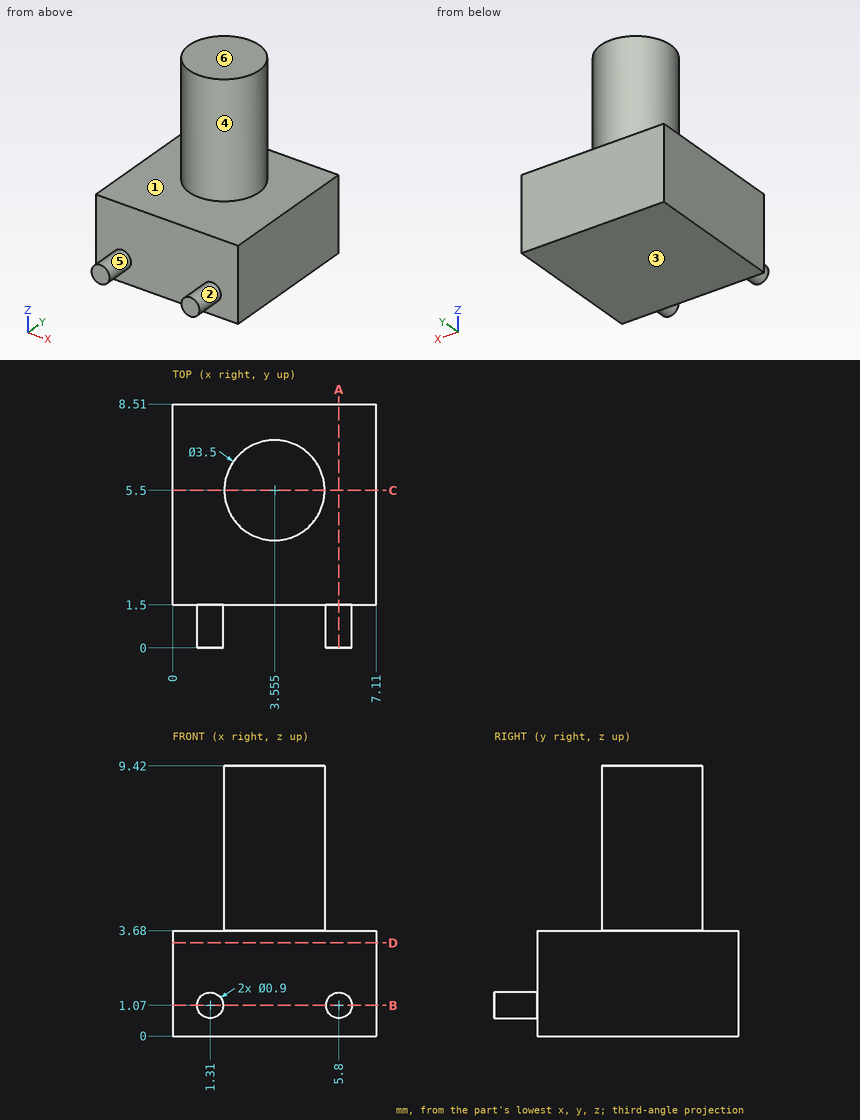
The figure shows three views and two pictorial views of one solid part (mm, origin at its lowest corner). Answer the questions. A direction names the side the tool comes from. Round coordinates to 2 decimals unless told otherwise and drop trailing zeros. Write each loop counter-clockwise with the first axis right and the second up, starting at its lowest first coordinate (ties: lowest second). Pieces come first, ordered by that corner, then holes. Notation, with made-up numbers: M 85.5,45.25 L 120.5,45.25 A16 ccw 120.5,76.25 Z; hole C 59.5,-7 d2. An arc over 180 degrees is marked long. Write each question's results on one line, items separated by ' | '. Start each with the question number.
(1) The part is cut by section A-A, the plane x = 5.8. Write down the section's boundary in (y, z), and give its area (3 significant figures).
(2) The part is cut by section C-C, the plane y = 5.5. Write down the section's boundary in (x, z) (3 decimals).
(3) The part is cut by section B-B, the plane z = 1.07. Write down the section's boundary in (x, y).
(4) The part is cut by section D-D, the plane z = 3.25. Write down the section's boundary in (x, y).
(5) For the marked faces 1, 2 and 3, determine the directions among +Z, -Z, +X, -X, +Y, -Y from which every point of the face is accessible in a straight line to the end or side of a thin tool.
(6) Determine the mould class of the marked faces 4, 5 and 6 for opening direction X: +X half, -X half, draft (parallel to the pull), parting line (faces both ways), or undercut.
(7) Find the intervals of material crossed by line 1 (Z direction, x = 6.75, y = 2); line 2 (X direction, y = 5.5, z = 6.5) (3 decimals); line 3 (Y direction, x = 2.5, z = 6.75), in increasing order.
(8) Each of these flat-tipped pins is pushed along its axis until it touches: P1, Ø2, axis at x = 5.5, y = 3.5, coming from the +Z side; P2, Ø5, axis at y = 5, z = 7, coming from the +X side (3 decimals); P3, Ø3, axis at y = 2.5, z = 7, coming from the -X side. Where does it stop, or does it pass through?
Worked answers:
1) outline: M 0,0.62 L 1.5,0.62 L 1.5,0 L 8.51,0 L 8.51,3.68 L 1.5,3.68 L 1.5,1.52 L 0,1.52 Z | area: 27.1 mm²
2) outline: M 0,0 L 7.11,0 L 7.11,3.68 L 5.305,3.68 L 5.305,9.42 L 1.805,9.42 L 1.805,3.68 L 0,3.68 Z
3) outline: M 0,1.5 L 0.86,1.5 L 0.86,0 L 1.76,0 L 1.76,1.5 L 5.35,1.5 L 5.35,0 L 6.25,0 L 6.25,1.5 L 7.11,1.5 L 7.11,8.51 L 0,8.51 Z
4) outline: M 0,1.5 L 7.11,1.5 L 7.11,8.51 L 0,8.51 Z
5) face 1: +Z | face 2: -Y | face 3: -Z, +X, -X, +Y, -Y
6) face 4: parting line | face 5: undercut | face 6: draft
7) line 1: z = 0 to 3.68 | line 2: x = 1.805 to 5.305 | line 3: y = 4.1 to 6.9
8) P1: stops at z = 3.68 | P2: stops at x = 5.305 | P3: stops at x = 2.65
